CAD build for the part. Positions are in the model's coordinates, mm. Coordinates: 2 decimals unless noted, no trailing zeros. Loops run counter-clockwise (first coordinate to the right, second up) from the corner with the lowest first, then second, coordinate; pieces in that order, holes last.
1) Saw through at C-C, the plane x = -13.5. Write the cut outline in (y, z).
2) Saw through at A-A, the plane y = 0.45. Write the cut outline in (x, z), and give its area (3 significant figures).
3) Wall check: line 1 along Z through (x, y) = (9, 0.95); line 2 along X through (y, z) = (0.3, -0.5); line 3 along X through (y, z) = (0.65, -24). Give the ranges that are in metal, low to high.
4) Saw through at B-B, the plane z = 14. Write the cut outline in (x, y).
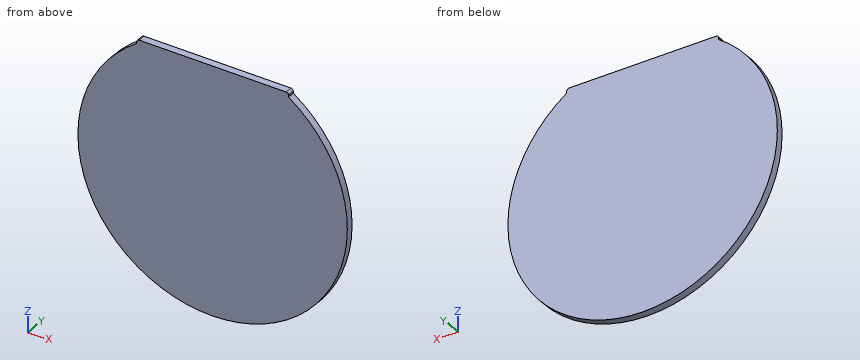
```python
from build123d import *

# Parameters (mm, degrees)
BOSS_EXTRUDE1_DEPTH = 1.5
FILLET1_R           = 0.5


with BuildPart() as part:
    # Sketch1 → Boss-Extrude1 (new body)
    with BuildSketch(Plane(origin=(0, 0, 0), x_dir=(1, 0, 0), z_dir=(0, 1, 0))):
        with BuildLine():
            Line((-15.5, -23.58495283), (15.5, -23.58495283))
            Line((15.5, -23.58495283), (15.5, -22.715633383))
            ThreePointArc((15.5, -22.715633383), (0, 27.5), (-15.5, -22.715633383))
            Line((-15.5, -22.715633383), (-15.5, -23.58495283))
        make_face()
    extrude(amount=BOSS_EXTRUDE1_DEPTH)

    # Fillet1
    fillet1_edges = [part.edges().sort_by_distance(p)[0] for p in [
        (15.5, 0.75, 23.58495283),
        (-15.5, 0.75, 23.58495283),
    ]]
    fillet(fillet1_edges, radius=FILLET1_R)


solid = part.part
```
Data:
1. outline: (0, -23.96) - (1.5, -23.96) - (1.5, 23.58) - (0, 23.58) - close
2. outline: (-15.5, 22.72) arc R27.5 ccw (long way) to (15.5, 22.72) - (15.5, 23.08) arc R0.5 ccw to (15, 23.58) - (-15, 23.58) arc R0.5 ccw to (-15.5, 23.08) - close
2. area: 2,300 mm2
3. line 1: z = -25.99 to 23.58
3. line 2: x = -27.5 to 27.5
3. line 3: x = -13.43 to 13.43
4. outline: (-23.67, 0) - (23.67, 0) - (23.67, 1.5) - (-23.67, 1.5) - close
